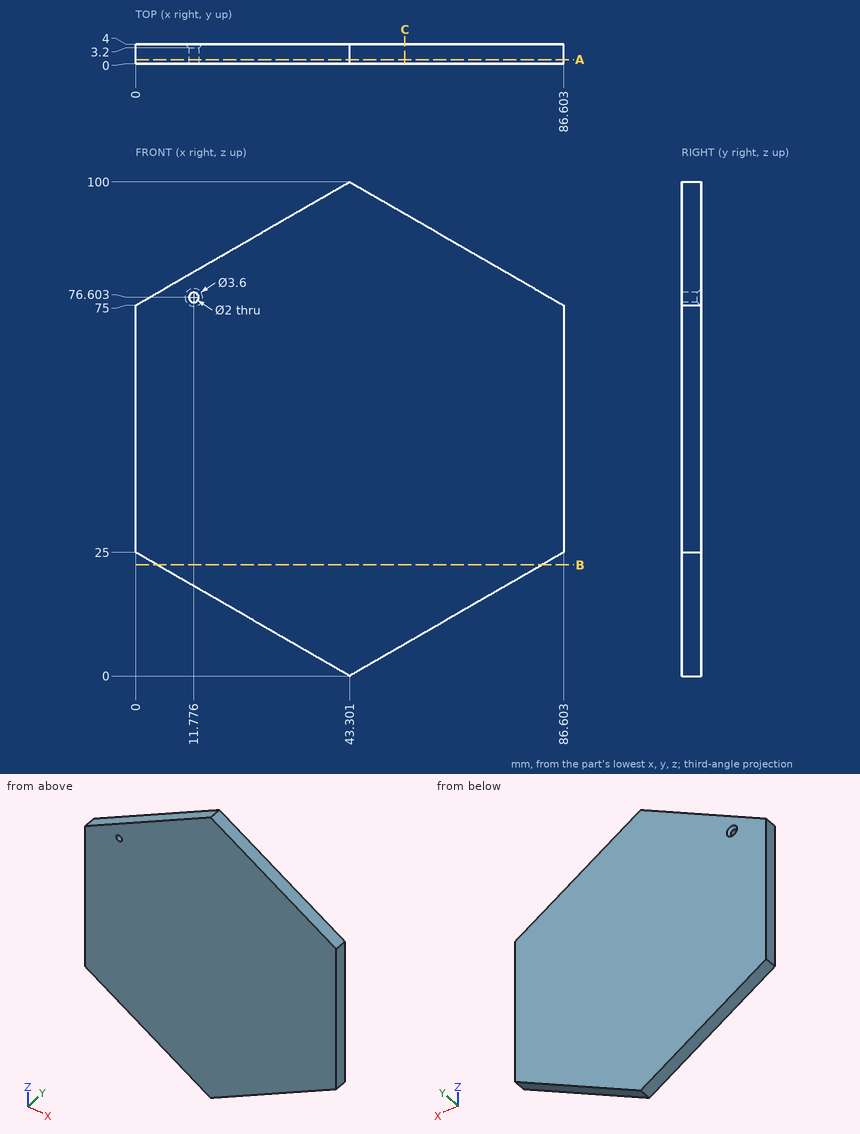
Verification items for this drawing (mm, ordinates from the low corner). Round coordinates to 2 decimals unless told otherwise and drop trailing zeros. Order: outer loops, then holes, each group sorted by start corner. A loop starts at its lowest first (then second) coordinate and runs counter-clockwise, first axis right, second up. Notation, with made-up numbers: (46.5, 67) -> (92.5, 67) arc R16 cw to (92.5, 72) -> close; hole circle Ø5 at (60.25, 22.25). An arc over 180 degrees is marked (long way). Use one line per item in the form item = value.
1. Cross-section at C-C, the plane x = 54.5. Enter the section's corners in (y, z) (1 decimal).
Working result:
outline = (0, 6.5) -> (4, 6.5) -> (4, 93.5) -> (0, 93.5) -> close
2. Cross-section at B-B, the plane z = 22.5. Enter the section's corners in (x, y), plus the area to 3 significant figures.
Working result:
outline = (4.33, 0) -> (82.27, 0) -> (82.27, 4) -> (4.33, 4) -> close
area = 312 mm^2
3. Cross-section at A-A, the plane y = 0.85. Enter the section's corners in (x, z), plus the area to 3 significant figures.
Working result:
outline = (0, 25) -> (43.3, 0) -> (86.6, 25) -> (86.6, 75) -> (43.3, 100) -> (0, 75) -> close; hole circle Ø2 at (11.78, 76.6)
area = 6,490 mm^2
4. Scan lines: line 1 along Z through (x, y) = (12.5, 0.4) (1 decimal); line 2 along Z through (x, y) = (77.5, 1.25) (1 decimal); line 3 along Z through (x, y) = (21.5, 2.9) (1 decimal). Record each from-to range of solid material in increasing order. Write a range as from..to.
Working result:
line_1 = 17.8..75.9, 77.3..82.2
line_2 = 19.7..80.3
line_3 = 12.6..87.4
5. Go/stop test with a flat-tipped pin: pin 1 (2 mm diameter, centred on y = 0.5, z = 36, fed in from -X). Record where the tip stops, or that it passes through.
Working result:
pin_1 = 0
